Source: CAD feature listing. Evaluate the final solid. Frame: model axes, mm. Face numbers are marked on the shaded views. Give positions to 0.01 mm unless a question says otherwise; leave off trailing zeros. Put each result on its own line as item: value.
```python
from build123d import *

# Parameters (mm, degrees)
SKETCH1_W             = 762
SKETCH1_H             = 177.8
BOSS_EXTRUDE1_DEPTH   = 3.175
BOSS_EXTRUDE1_2_DEPTH = 3.175
SKETCH2_W             = 12.7
SKETCH2_H             = 25.198455275
SKETCH2_W_2           = 12.652375
SKETCH2_H_2           = 20.883441122
BOSS_EXTRUDE2_DEPTH   = 3.175
SKETCH3_R             = 2.413
CUT_EXTRUDE1_DEPTH    = 392.247096756


with BuildPart() as part:
    # Sketch1 → Boss-Extrude1 (new body)
    with BuildSketch(Plane.XY):
        Rectangle(SKETCH1_W, SKETCH1_H)
        with BuildLine():
            Line((-98.898075, -39.835315096), (-126.47295, -39.835315096))
            Line((-126.47295, -39.835315096), (-112.69345, 25.109309904))
            Line((-112.69345, 25.109309904), (-125.39345, 25.109309904))
            Line((-125.39345, 25.109309904), (-127.981075, 12.822059904))
            Line((-127.981075, 12.822059904), (-155.55595, 12.822059904))
            Line((-155.55595, 12.822059904), (-153.4922, 24.061559904))
            add(Edge.make_bspline(
                [(-153.4922, 24.061559904), (-153.114009041, 25.826838845), (-152.107111159, 28.330892524), (-150.018844738, 31.208697921), (-148.110526346, 33.000169059), (-145.952379495, 34.474150169), (-142.756393957, 35.899752111), (-140.131656162, 36.29243254), (-138.3792, 36.285309904)],
                knots=[0, 0, 0, 0, 0.256781092, 0.379270402, 0.504103305, 0.627938883, 0.75015623, 1, 1, 1, 1], degree=3))
            Line((-138.3792, 36.285309904), (-82.9437, 36.285309904))
            Line((-82.9437, 36.285309904), (-98.898075, -39.835315096))
        make_face(mode=Mode.SUBTRACT)
        with BuildLine():
            Line((-27.695525, -39.914690096), (-69.478525, -39.914690096))
            add(Edge.make_bspline(
                [(-69.478525, -39.914690096), (-70.378419778, -39.890724934), (-71.704855295, -39.834182103), (-73.367269691, -39.428139507), (-74.4978262, -39.054475963), (-75.523062052, -38.544153837), (-76.467505593, -37.933458517), (-77.303402375, -37.199179804), (-78.055411522, -36.372825302), (-78.694544311, -35.450572391), (-79.192076882, -34.444787097), (-79.609552025, -33.388191923), (-79.846110554, -32.250761591), (-80.002676754, -31.050614438), (-79.979776999, -29.310279003), (-79.819248509, -27.981119838), (-79.62265, -27.087690096)],
                knots=[0, 0, 0, 0, 0.140211227, 0.204364429, 0.265147851, 0.324658092, 0.381613589, 0.439257912, 0.496831965, 0.554704074, 0.612744983, 0.670716103, 0.730497823, 0.792544611, 0.858256418, 1, 1, 1, 1], degree=3))
            Line((-79.62265, -27.087690096), (-68.8594, 23.871059904))
            add(Edge.make_bspline(
                [(-68.8594, 23.871059904), (-68.462815939, 25.643057301), (-67.505422501, 28.206697467), (-65.384523981, 31.101105561), (-63.495671972, 32.940400282), (-61.340054695, 34.44245551), (-58.13780239, 35.889129542), (-55.506378001, 36.299143413), (-53.7464, 36.285309904)],
                knots=[0, 0, 0, 0, 0.257514098, 0.38084006, 0.505341434, 0.629198731, 0.750909855, 1, 1, 1, 1], degree=3))
            Line((-53.7464, 36.285309904), (-11.9634, 36.285309904))
            add(Edge.make_bspline(
                [(-11.9634, 36.285309904), (-10.951206406, 36.265095396), (-9.472034389, 36.198930496), (-7.598624422, 35.809565279), (-6.362047596, 35.393919508), (-5.226995923, 34.884334314), (-4.209362568, 34.252182113), (-3.309508264, 33.490388009), (-2.517821843, 32.639137402), (-1.849309358, 31.697562392), (-1.305537987, 30.689972363), (-0.888869485, 29.624844052), (-0.618683845, 28.492151076), (-0.479667068, 27.309465242), (-0.461795302, 25.606385314), (-0.640427295, 24.310954775), (-0.8509, 23.442434904)],
                knots=[0, 0, 0, 0, 0.150988733, 0.2194496, 0.284234088, 0.344880513, 0.404348422, 0.461954929, 0.519942779, 0.577007859, 0.633416367, 0.690044579, 0.746804204, 0.806324292, 0.867001421, 1, 1, 1, 1], degree=3))
            Line((-0.8509, 23.442434904), (-11.61415, -27.532190096))
            add(Edge.make_bspline(
                [(-11.61415, -27.532190096), (-11.987729804, -29.240567183), (-13.011146829, -31.705361087), (-15.153529873, -34.541520304), (-16.794536644, -36.112916543), (-18.285460276, -37.193344942), (-19.453657133, -37.934268454), (-20.694525744, -38.533784236), (-21.977681798, -39.054718418), (-23.334799484, -39.420538407), (-25.229442597, -39.826610751), (-26.705398031, -39.890467006), (-27.695525, -39.914690096)],
                knots=[0, 0, 0, 0, 0.238595474, 0.358933013, 0.483744219, 0.547388327, 0.610400664, 0.672497519, 0.7354808, 0.799354582, 0.864312251, 1, 1, 1, 1], degree=3))
        make_face(mode=Mode.SUBTRACT)
        with BuildLine():
            Line((42.8244, 36.285309904), (33.982025, -5.370690096))
            Line((33.982025, -5.370690096), (46.6344, -5.370690096))
            Line((46.6344, -5.370690096), (55.476775, 36.285309904))
            Line((55.476775, 36.285309904), (83.099275, 36.285309904))
            Line((83.099275, 36.285309904), (67.129025, -39.914690096))
            Line((67.129025, -39.914690096), (39.55415, -39.914690096))
            Line((39.55415, -39.914690096), (44.50715, -16.546690096))
            Line((44.50715, -16.546690096), (16.88465, -16.546690096))
            add(Edge.make_bspline(
                [(16.88465, -16.546690096), (15.97397184, -16.566803466), (14.654465721, -16.442849527), (12.969679896, -16.084165205), (11.848493473, -15.685263746), (10.814508554, -15.187184105), (9.866010852, -14.585783269), (9.028628771, -13.846530809), (8.274838484, -13.021287426), (7.643672663, -12.100509132), (7.126661545, -11.105170566), (6.749218091, -10.040732714), (6.496795936, -8.910572682), (6.345702881, -7.71402033), (6.366723836, -5.974283719), (6.528488375, -4.644730591), (6.72465, -3.751440096)],
                knots=[0, 0, 0, 0, 0.141055917, 0.205006137, 0.266817017, 0.325211674, 0.382839171, 0.440466668, 0.498023916, 0.555879133, 0.613172181, 0.671613009, 0.730576487, 0.792605165, 0.858297791, 1, 1, 1, 1], degree=3))
            Line((6.72465, -3.751440096), (15.186025, 36.285309904))
            Line((15.186025, 36.285309904), (42.8244, 36.285309904))
        make_face(mode=Mode.SUBTRACT)
        with BuildLine():
            Line((116.900325, -28.738690096), (157.1752, -28.738690096))
            Line((157.1752, -28.738690096), (155.000325, -39.914690096))
            Line((155.000325, -39.914690096), (87.1347, -39.914690096))
            Line((87.1347, -39.914690096), (91.5797, -17.800815096))
            add(Edge.make_bspline(
                [(91.5797, -17.800815096), (91.970731994, -16.024994145), (92.943076158, -13.475373477), (95.037802627, -10.562190947), (96.626678786, -9.030826572), (98.04129727, -7.984571288), (99.140031696, -7.270780811), (100.298338787, -6.689209352), (101.495760204, -6.213878956), (102.724230789, -5.824722646), (104.446719435, -5.462579309), (105.778975302, -5.364834977), (106.676825, -5.370690096)],
                knots=[0, 0, 0, 0, 0.257512197, 0.380397285, 0.505435299, 0.568066423, 0.629375226, 0.690688606, 0.751204987, 0.811628551, 0.872900724, 1, 1, 1, 1], degree=3))
            Line((106.676825, -5.370690096), (134.5057, -5.370690096))
            Line((134.5057, -5.370690096), (141.20495, 25.109309904))
            Line((141.20495, 25.109309904), (128.50495, 25.109309904))
            Line((128.50495, 25.109309904), (125.917325, 12.822059904))
            Line((125.917325, 12.822059904), (98.34245, 12.822059904))
            Line((98.34245, 12.822059904), (100.4062, 24.061559904))
            add(Edge.make_bspline(
                [(100.4062, 24.061559904), (100.784390959, 25.826838845), (101.791288841, 28.330892524), (103.879555262, 31.208697921), (105.787873654, 33.000169059), (107.946020505, 34.474150169), (111.142006043, 35.899752111), (113.766743838, 36.29243254), (115.5192, 36.285309904)],
                knots=[0, 0, 0, 0, 0.256781092, 0.379270402, 0.504103305, 0.627938883, 0.75015623, 1, 1, 1, 1], degree=3))
            Line((115.5192, 36.285309904), (157.3022, 36.285309904))
            add(Edge.make_bspline(
                [(157.3022, 36.285309904), (158.313404759, 36.262334312), (159.795356307, 36.203930585), (161.662996805, 35.803296989), (162.915290146, 35.415626042), (164.04161951, 34.88092493), (165.077257642, 34.2714369), (165.971103509, 33.504855616), (166.764093589, 32.655469989), (167.431275951, 31.713004044), (167.97575393, 30.713137791), (168.378470101, 29.644245275), (168.643854599, 28.518162675), (168.787088091, 27.33606961), (168.802987002, 25.638048994), (168.625616664, 24.342751641), (168.4147, 23.474184904)],
                knots=[0, 0, 0, 0, 0.151086534, 0.219591746, 0.284173196, 0.345905024, 0.404997354, 0.462641174, 0.520666586, 0.577768628, 0.634213675, 0.689860087, 0.747422966, 0.80619884, 0.866915273, 1, 1, 1, 1], degree=3))
            Line((168.4147, 23.474184904), (162.60445, -4.195940096))
            add(Edge.make_bspline(
                [(162.60445, -4.195940096), (162.222762109, -5.895405939), (161.212748067, -8.357775045), (159.060484323, -11.176073851), (157.423570654, -12.736969042), (155.946992387, -13.829638667), (154.777335182, -14.570198188), (153.527544548, -15.162182906), (152.245499952, -15.683808477), (150.890272205, -16.057436379), (148.993426207, -16.45398034), (147.513691649, -16.524751422), (146.523075, -16.546690096)],
                knots=[0, 0, 0, 0, 0.238188423, 0.358091, 0.48305048, 0.546187513, 0.609274708, 0.67209543, 0.735153534, 0.798406705, 0.864151056, 1, 1, 1, 1], degree=3))
            Line((146.523075, -16.546690096), (119.67845, -16.546690096))
            Line((119.67845, -16.546690096), (116.900325, -28.738690096))
        make_face(mode=Mode.SUBTRACT)
    extrude(amount=BOSS_EXTRUDE1_DEPTH)



with BuildPart() as body_2:
    # Sketch1 → Boss-Extrude1 2 (new body)
    with BuildSketch(Plane.XY):
        Polygon((-40.76065, 25.109309904), (-52.365275, -28.738690096), (-39.7129, -28.738690096), (-28.06065, 25.109309904), align=None)
    extrude(amount=BOSS_EXTRUDE1_2_DEPTH)


with BuildPart() as part_1:
    add(part.part)

    add(body_2.part)  # Boss-Extrude2 merges body 2
    # Sketch2 → Boss-Extrude2 (add)
    with BuildSketch(Plane.XY.offset(3.175)):
        with Locations((-34.41065, 37.708537542)):
            Rectangle(SKETCH2_W, SKETCH2_H)
        with Locations((-46.0390875, -39.180410657)):
            Rectangle(SKETCH2_W_2, SKETCH2_H_2)
    extrude(amount=-BOSS_EXTRUDE2_DEPTH)

    # Sketch3 → Cut-Extrude1 (cut, through all)
    with BuildSketch(Plane.XY.offset(3.175)):
        with Locations((-368.3, 76.2)):
            Circle(SKETCH3_R)
        with Locations((-368.3, 38.1)):
            Circle(SKETCH3_R)
        with Locations((-368.3, 0)):
            Circle(SKETCH3_R)
        with Locations((-368.3, -38.1)):
            Circle(SKETCH3_R)
        with Locations((-368.3, -76.2)):
            Circle(SKETCH3_R)
        with Locations(Location((368.3, -76.2, 0), (0, 0, 180))):
            Circle(SKETCH3_R)
        with Locations(Location((368.3, -38.1, 0), (0, 0, 180))):
            Circle(SKETCH3_R)
        with Locations(Location((368.3, 0, 0), (0, 0, 180))):
            Circle(SKETCH3_R)
        with Locations(Location((368.3, 38.1, 0), (0, 0, 180))):
            Circle(SKETCH3_R)
        with Locations(Location((368.3, 76.2, 0), (0, 0, 180))):
            Circle(SKETCH3_R)
    extrude(amount=-CUT_EXTRUDE1_DEPTH, mode=Mode.SUBTRACT)


solid = part_1.part
```
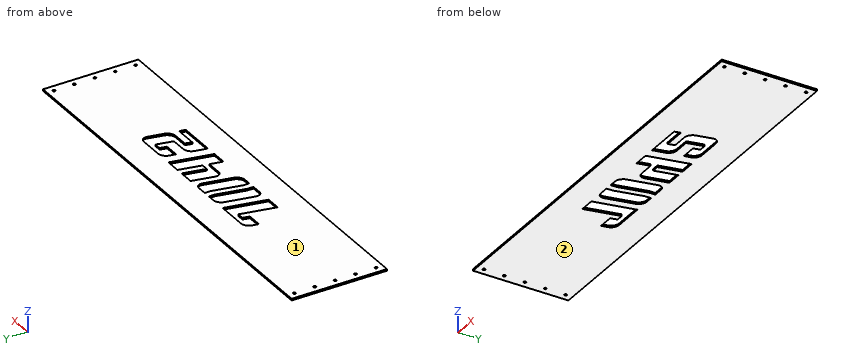
(1) Draft query along Z for the marked faces 1 and 2. Return one class per face: released by +Z, released by -Z, zero draft, split by the parting line, or undercut.
Calculated:
face 1: released by +Z
face 2: released by -Z
(2) Section A-A on z = 2.45. Give the number of separate pieces and of enclosed holes in the cut face, then the cut area to 3 significant figures.
Calculated:
separate pieces: 1
enclosed holes: 15
area: 121,000 mm²
(3) Line query: probe 1 along Y at (x, z) = (368.3, 1.9); probe 2 along X at (y, z) = (-75, 2.95); probe 3 along X at (y, z) = (-7, 1). Output: solid intervals per line, ascending. Write a range as from..to.
Calculated:
probe 1: y = -88.9..-78.61, -73.79..-40.51, -35.69..-2.41, 2.41..35.69, 40.51..73.79, 78.61..88.9
probe 2: x = -381..-370.39, -366.21..366.21, 370.39..381
probe 3: x = -381..-119.51, -92.02..-75.38, -47.68..-35.01, -7.28..6.36, 74.03..99.69, 161.68..381
